Autodesk Inventor part; units mm, degrees
ref_plane "YZ Plane" through (0, 0, 0) normal (1, 0, 0) x (0, 1, 0)
ref_plane "XZ Plane" through (0, 0, 0) normal (0, 1, 0) x (-1, 0, 0)
ref_plane "XY Plane" through (0, 0, 0) normal (0, 0, 1) x (1, 0, 0)
sketch "Sketch1" plane through (0, 0, 0) normal (0, 1, 0) x (-1, 0, 0)
  line L0 (55, 0) -> (-69, 0) construction
  line L1 (0, 72) -> (0, -101) construction
  line L2 (35, 78.5) -> (-35, 78.5)
  line L3 (-35, 78.5) -> (-35, -78.5)
  line L4 (-35, -78.5) -> (35, -78.5)
  line L5 (35, -78.5) -> (35, 78.5)
  line L6 (35, 78.5) -> (-35, -78.5) construction
  line L7 (-35, 78.5) -> (35, -78.5) construction
  line L8 (37, 80.5) -> (-37, 80.5)
  line L9 (-37, 80.5) -> (-37, -80.5)
  line L10 (-37, -80.5) -> (37, -80.5)
  line L11 (37, -80.5) -> (37, 80.5)
  line L12 (37, 80.5) -> (-37, -80.5) construction
  line L13 (-37, 80.5) -> (37, -80.5) construction
  circle A0 centre (20, -70) radius 1.6
  circle A1 centre (20, -70) radius 2.75
  circle A2 centre (-14, -70) radius 1.6
  circle A3 centre (-14, -70) radius 2.75
  circle A4 centre (20, 70) radius 1.6
  circle A5 centre (20, 70) radius 2.75
  circle A6 centre (-14, 70) radius 1.6
  circle A7 centre (-14, 70) radius 2.75
  line L14 (35, 78.5) -> (30, 78.5)
  line L15 (30, 78.5) -> (30, 73.5)
  line L16 (30, 73.5) -> (35, 73.5)
  line L17 (35, 73.5) -> (35, 78.5)
  line L18 (-35, 78.5) -> (-30, 78.5)
  line L19 (-30, 78.5) -> (-30, 73.5)
  line L20 (-30, 73.5) -> (-35, 73.5)
  line L21 (-35, 73.5) -> (-35, 78.5)
  line L22 (35, -78.5) -> (30, -78.5)
  line L23 (30, -78.5) -> (30, -73.5)
  line L24 (30, -73.5) -> (35, -73.5)
  line L25 (35, -73.5) -> (35, -78.5)
  line L26 (-35, -78.5) -> (-30, -78.5)
  line L27 (-30, -78.5) -> (-30, -73.5)
  line L28 (-30, -73.5) -> (-35, -73.5)
  line L29 (-35, -73.5) -> (-35, -78.5)
  line L30 (40, -5) -> (30, -5)
  line L31 (30, -5) -> (30, 5)
  line L32 (30, 5) -> (40, 5)
  line L33 (40, 5) -> (40, -5)
  line L34 (40, -5) -> (30, 5) construction
  line L35 (30, -5) -> (40, 5) construction
  line L36 (-30, -5) -> (-40, -5)
  line L37 (-40, -5) -> (-40, 5)
  line L38 (-40, 5) -> (-30, 5)
  line L39 (-30, 5) -> (-30, -5)
  line L40 (-30, -5) -> (-40, 5) construction
  line L41 (-40, -5) -> (-30, 5) construction
  point P0 (0, 0)
  point P1 (35, 0)
  point P2 (-35, 0)
  point P3 (-35, 5)
  point P4 (-35, -5)
  point P5 (35, -5)
  point P6 (35, 5)
  dimension "d0" = 70
  dimension "d1" = 157
  dimension "d2" = 74
  dimension "d3" = 161
  dimension "d4" = 3.2
  dimension "d5" = 17
  dimension "d6" = 70
  dimension "d7" = 5.5
  dimension "d8" = 3.2
  dimension "d9" = 5.5
  dimension "d10" = 34
  dimension "d11" = 5
  dimension "d12" = 5
  dimension "d13" = 5
  dimension "d14" = 5
  dimension "d15" = 5
  dimension "d16" = 5
  dimension "d17" = 5
extrude "Extrusion1" add sketch "Sketch1" along normal blind 2 contours L15 L16 L5 L32 L31 L30 L24 L23 L4 L27 L28 L3 L36 L39 L38 L20 L19 L2 | L5 L30 L31 L32 | L38 L39 L36 L3 | A1 | A3 | A5 | A7
extrude "Extrusion2" add sketch "Sketch1" along normal blind 25 contours L5 L16 L15 L2 | L19 L20 L3 L2 | L5 L30 L31 L32 | L5 L4 L23 L24 | L38 L39 L36 L3 | L28 L27 L4 L3
extrude "Extrusion3" add sketch "Sketch1" along normal blind 30 contours L2 L3 L38 L9 L8 L11 L32 L5 | L32 L11 L30 L5 | L30 L11 L10 L9 L36 L3 L4 L5 | L3 L36 L9 L38
properties part number "Mounting Master_3DPrint"
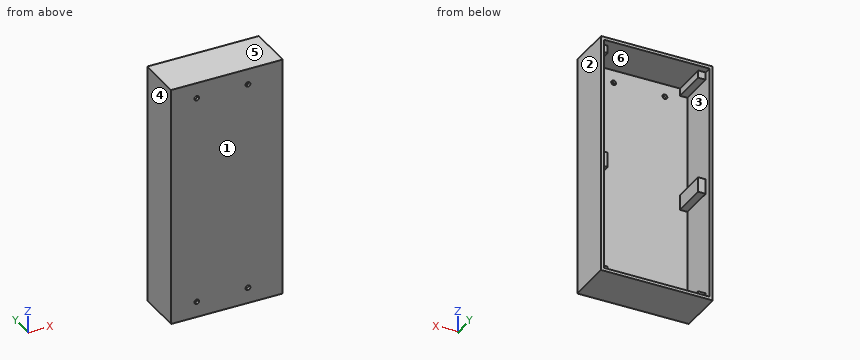
Here's how the part is built. I have some questions about the finished solid (model axes, mm). Face numbers are marked on the shaded views. A direction names the side the tool comes from. Round coordinates to 2 decimals unless told otherwise and drop trailing zeros. Order: outer loops, then holes, each group sorted by start corner. A loop starts at its lowest first (then second) coordinate and runs counter-clockwise, first axis right, second up. Notation, with made-up numbers: (-32.75, -39) -> (-25.75, -39) arc R32 cw to (-25.75, -8) -> close; hole circle Ø9 at (72, 49). An arc over 180 degrees is marked (long way). Use a Markdown table: item, result. Add a question column.
(1) Suppose I cut it at D-D, the plane x = 2. Please give me the cut outline in (y, z).
(2) For the marked faces 5 and 6, which set-ups out of +Z, -Z, +X, -X, +Y, -Y let a thin tool reach every point of the face, with its end or its side?
(3) Suppose I cut it at A-A, the plane x = 14. Please give me the cut outline in (y, z).
(4) For pin 1 Ø10 at (x, z) = (8, -18) entering from -Y; pin 2 Ø4 at (x, z) = (14, 70) entering from +Y; pin 3 Ø2.5 at (x, z) = (-32.5, -1) entering from +Y, each with a flat end and sliding along its axis, tell me the tip position at first contact or that it passes through.
(5) I need wall thicknesses on line 1 along Z through (x, y) = (14, 1); line 2 along X through (y, z) = (0.6, 70); line 3 along Z through (x, y) = (31.5, 22). Which ranges of each line are inside material? Lowest first, please.
(6) If we mould it in two halves opening along X, with no side actions, what happens to the marked faces 1, 2, 3 and 4? For each: released by +X, released by -X, zero draft, split by the parting line, or undercut.
(7) Suppose I cut it at B-B, the plane z = 70. Please give me the cut outline in (x, y), and give its area (3 significant figures).
(8) Suppose I cut it at C-C, the plane y = 8. Please give me the cut outline in (x, z).
Verdict:
| question | item | result |
|---|---|---|
| 1 | outline | (0, -80.5) -> (30, -80.5) -> (30, -78.5) -> (2, -78.5) -> (2, 78.5) -> (30, 78.5) -> (30, 80.5) -> (0, 80.5) -> close |
| 2 | face 5 | +Z, +X, -X, +Y, -Y |
| 2 | face 6 | +Y |
| 3 | outline | (0, -80.5) -> (30, -80.5) -> (30, -78.5) -> (2, -78.5) -> (2, -71.6) -> (0, -71.6) -> close; (0, -68.4) -> (2, -68.4) -> (2, 68.4) -> (0, 68.4) -> close; (0, 71.6) -> (2, 71.6) -> (2, 78.5) -> (30, 78.5) -> (30, 80.5) -> (0, 80.5) -> close |
| 4 | pin 1 | y = 0 |
| 4 | pin 2 | y = 2 |
| 4 | pin 3 | y = 25 |
| 5 | line 1 | -80.5 to -71.6, -68.4 to 68.4, 71.6 to 80.5 |
| 5 | line 2 | -37 to -21.6, -18.4 to 12.4, 15.6 to 37 |
| 5 | line 3 | -80.5 to -73.5, -5 to 5, 73.5 to 80.5 |
| 6 | face 1 | zero draft |
| 6 | face 2 | released by +X |
| 6 | face 3 | undercut |
| 6 | face 4 | released by -X |
| 7 | outline | (-37, 0) -> (-21.6, 0) -> (-21.6, 2) -> (-35, 2) -> (-35, 30) -> (-37, 30) -> close; (-18.4, 0) -> (12.4, 0) -> (12.4, 2) -> (-18.4, 2) -> close; (15.6, 0) -> (37, 0) -> (37, 30) -> (35, 30) -> (35, 2) -> (15.6, 2) -> close |
| 7 | area | 247 mm2 |
| 8 | outline | (-37, -80.5) -> (37, -80.5) -> (37, 80.5) -> (-37, 80.5) -> close; hole (-35, -73.5) -> (-30, -73.5) -> (-30, -78.5) -> (30, -78.5) -> (30, -73.5) -> (35, -73.5) -> (35, -5) -> (30, -5) -> (30, 5) -> (35, 5) -> (35, 73.5) -> (30, 73.5) -> (30, 78.5) -> (-30, 78.5) -> (-30, 73.5) -> (-35, 73.5) -> (-35, 5) -> (-30, 5) -> (-30, -5) -> (-35, -5) -> close |
